Geometry check sheet. Reference: the model listing, model coordinates, mm. Give positions to 0.01 mm unless a question says otherwise; leave off trailing zeros. Loops run counter-clockwise (first coordinate to the right, second up) from the corner with the lowest first, then second, coordinate; pieces in that order, holes last.
1. Cross-section at A-A, the plane y = 0. Record the cut outline in (x, z).
2. Material ranges on L1, parallel to X at y = -2.25, z = -2.5; L2, parallel to Z at x = -121.5, y = 2.25; L3, parallel to Z at x = -101.5, y = 1.25, recorded low to high.
3. Cross-section at B-B, the plane x = -217.5. Record the cut outline in (y, z).
4. Go/stop test with flat-tipped pins: pin 1 Ø1 at (x, y) = (-83.5, 5) entering from -Z; pin 2 Ø1 at (y, z) = (-3.5, 1.5) entering from -X; pin 3 Ø8 at (x, y) = (-91.5, -0.5) entering from +Z. Record where each tip stops, or that it passes through.
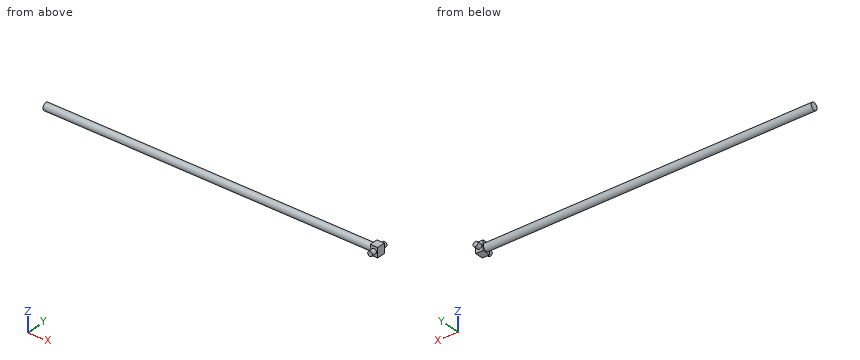
from build123d import *

# Parameters (mm, degrees)
F0_W     = 6
F0_H     = 8
F1_DEPTH = 7.4
F2_W     = 6
F2_H     = 8
F2_R     = 2
F3_DEPTH = 4
F4_W     = 6
F4_H     = 8
F4_R     = 2
F5_DEPTH = 4
F6_R     = 3
F7_DEPTH = 167.74
F8_R     = 3
F9_DEPTH = 100


with BuildPart() as f1:
    # F0 (on Front) → F1 (new body, symmetric)
    with BuildSketch(Plane.XZ):
        Rectangle(F0_W, F0_H)
    extrude(amount=F1_DEPTH, both=True)

    # F2 (on face) → F3 (cut)
    with BuildSketch(Plane.XZ.offset(7.4)):
        Rectangle(F2_W, F2_H)
        Circle(F2_R, mode=Mode.SUBTRACT)
    extrude(amount=-F3_DEPTH, mode=Mode.SUBTRACT)

    # F4 (on face) → F5 (cut)
    with BuildSketch(Plane(origin=(0, 7.4, 0), x_dir=(-1, 0, 0), z_dir=(0, 1, 0))):
        Rectangle(F4_W, F4_H)
        Circle(F4_R, mode=Mode.SUBTRACT)
    extrude(amount=-F5_DEPTH, mode=Mode.SUBTRACT)

    # F6 (on face) → F7 (join)
    with BuildSketch(Plane(origin=(-3, 0, 0), x_dir=(0, -1, 0), z_dir=(-1, 0, 0))):
        Circle(F6_R)
    extrude(amount=F7_DEPTH)

    # F8 (on face) → F9 (join)
    with BuildSketch(Plane(origin=(-170.74, 0, 0), x_dir=(0, -1, 0), z_dir=(-1, 0, 0))):
        Circle(F8_R)
    extrude(amount=F9_DEPTH)


solid = f1.part
Result:
1. outline: (-270.74, -3) - (-3, -3) - (-3, -4) - (3, -4) - (3, 4) - (-3, 4) - (-3, 3) - (-270.74, 3) - close
2. L1: x = -3 to 3
2. L2: z = -1.98 to 1.98
2. L3: z = -2.73 to 2.73
3. outline: circle Ø6 at (0, 0)
4. pin 1: passes through
4. pin 2: stops at x = -3
4. pin 3: stops at z = 3
